Design review of the part built by this model. Coordinates are the model's own, in mm. Face numbers are marked on the shaded views. A direction names the side the tool comes from. Give positions to 0.01 mm unless a question says otherwise; leave off trailing zeros. Order: outer loops, then holes, each group sorted by start corner. A loop starts at its lowest first (then second) coordinate and runs counter-clockwise, first axis right, second up. Notation, with made-up numbers: (2, 11) -> (50, 11) arc R14 ccw to (50, 33) -> close; hole circle Ø6 at (31, 48.5). An arc over 180 degrees is marked (long way). One line per item, written item: value. Start each with the question number.
1) Consider section C-C (z = 31.5). State the section outline as (x, y) points, plus the area to 3 significant figures.
2) For pin 1 (2 mm diameter, centred on y = 8.5, z = 34.5, fed in from +X); pin 2 (3 mm diameter, centred on x = -9, z = 31.5, fed in from -Y); pin 3 (3 mm diameter, centred on x = -6.5, y = 4.5, fed in from +Z), all flat-tipped, find the tip position at first contact; note any pin that passes through.
3) Consider section B-B (y = 0). State the section outline as (x, z) points, plus the area to 3 significant figures.
4) Consider section A-A (x = 0). State the section outline as (y, z) points, plus the area to 3 significant figures.
5) Consider section D-D (x = 10.75). State the section outline as (y, z) points.
6) The part is to be moulded in two halves that separate along X. For the marked faces 1, 2 and 3, say which applies: released by +X, released by -X, zero draft, split by the parting line, or undercut.
7) Tool access review of the marked faces 4, 5 and 6: name each direction out of +Z, -Z, +X, -X, +Y, -Y from which nothing blocks a thin tool from reaching the whole face with its end or side.
8) Wall thickness on line 1 along Y through (x, z) = (0, 34); line 2 along Z through (x, y) = (-1, -6.75); line 3 along Y through (x, z) = (6.75, 31.5): over which ranges is each line inside the solid? List them lowest first. Write a range as from..to.
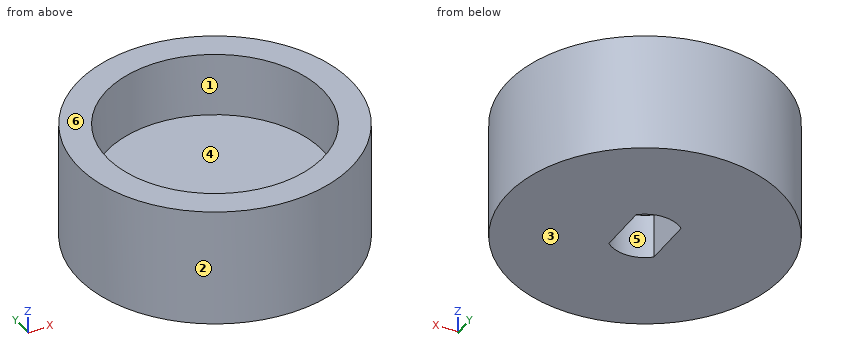
from build123d import *

# Parameters (mm, degrees)
BOX005_W          = 10
BOX005_H          = 10
BOX005_DEPTH      = 40
BOX004_W          = 10
BOX004_H          = 10
BOX004_DEPTH      = 40
CYLINDER011_R     = 3.7
CYLINDER011_DEPTH = 36.1
CYLINDER013_R     = 11.85
CYLINDER013_DEPTH = 100
CYLINDER012_R     = 15
CYLINDER012_DEPTH = 13


with BuildPart() as cube005:
    # Box005 → Box005 (new body)
    with BuildSketch(Plane(origin=(-1.85, -5, 5), x_dir=(1, 0, 0), z_dir=(0, 0, 1))):
        with Locations((5, 5)):
            Rectangle(BOX005_W, BOX005_H)
    extrude(amount=BOX005_DEPTH)


with BuildPart() as cube004:
    # Box004 → Box004 (new body)
    with BuildSketch(Plane(origin=(13.05, -5, -11), x_dir=(1, 0, 0), z_dir=(0, 0, 1))):
        with Locations((5, 5)):
            Rectangle(BOX004_W, BOX004_H)
    extrude(amount=BOX004_DEPTH)


with BuildPart() as drive001:
    # Cylinder011 → Cylinder011 (new body)
    with BuildSketch(Plane(origin=(10.6, 0, -9.2), x_dir=(1, 0, 0), z_dir=(0, 0, 1))):
        Circle(CYLINDER011_R)
    extrude(amount=CYLINDER011_DEPTH)

    # Cut005: cut Cube004
    add(cube004.part, mode=Mode.SUBTRACT)

    # Cut055: cut Cube005
    add(cube005.part, mode=Mode.SUBTRACT)


with BuildPart() as drive001_1:
    # Cut055 placement: moved
    add(drive001.part.moved(Location((-10.6, 0, 3))))


with BuildPart() as cylinder006:
    # Cylinder013 → Cylinder013 (new body)
    with BuildSketch(Plane.XY.offset(31)):
        Circle(CYLINDER013_R)
    extrude(amount=CYLINDER013_DEPTH)


with BuildPart() as winder_end_motor:
    # Cylinder012 → Cylinder012 (new body)
    with BuildSketch(Plane.XY.offset(25)):
        Circle(CYLINDER012_R)
    extrude(amount=CYLINDER012_DEPTH)

    # Cut054: cut Cylinder006
    add(cylinder006.part, mode=Mode.SUBTRACT)

    # Cut056: cut drive001
    add(drive001_1.part, mode=Mode.SUBTRACT)


solid = winder_end_motor.part
Checked values:
1. outline: circle Ø30 at (0, 0); hole circle Ø23.7 at (0, 0)
1. area: 266 mm^2
2. pin 1: stops at x = 12.99
2. pin 2: stops at y = -12.99
2. pin 3: stops at z = 31
3. outline: (-15, 25) -> (-2.45, 25) -> (-2.45, 29.9) -> (2.45, 29.9) -> (2.45, 25) -> (15, 25) -> (15, 38) -> (11.85, 38) -> (11.85, 31) -> (-11.85, 31) -> (-11.85, 38) -> (-15, 38) -> close
3. area: 200 mm^2
4. outline: (-15, 25) -> (-3.7, 25) -> (-3.7, 29.9) -> (3.7, 29.9) -> (3.7, 25) -> (15, 25) -> (15, 38) -> (11.85, 38) -> (11.85, 31) -> (-11.85, 31) -> (-11.85, 38) -> (-15, 38) -> close
4. area: 188 mm^2
5. outline: (-10.46, 25) -> (10.46, 25) -> (10.46, 38) -> (4.99, 38) -> (4.99, 31) -> (-4.99, 31) -> (-4.99, 38) -> (-10.46, 38) -> close
6. face 1: undercut
6. face 2: split by the parting line
6. face 3: zero draft
7. face 4: +Z
7. face 5: -Z
7. face 6: +Z, +X, -X, +Y, -Y
8. line 1: y = -15..-11.85, 11.85..15
8. line 2: z = 25..31
8. line 3: y = -13.4..-9.74, 9.74..13.4
